For this review, take the finished solid that the model builds, in its own axes (mm). A direction names the side the tool comes from. Coordinates: 2 decimals unless noted, no trailing zeros. Loops run counter-clockwise (first coordinate to the right, second up) from the corner with the lowest first, then second, coordinate; pieces in that order, holes last. Notation, with made-up numbers: (37.25, -29.5) - (44.25, -29.5) arc R18 cw to (44.25, -3.5) - close; hole circle Ø7 at (47.5, 46). An arc over 180 degrees is marked (long way). Answer as a JSON object with one key per item and string values. Group by question number.
Item 1: To check wall thickness, follow line 1 (Y direction, x = 2, z = 1.5); line 2 (X direction, y = 2, z = -0.75); line 3 (Z direction, x = 0, y = 2). State the ranges of each line that lie inside material, in increasing order.
Item 2: We need section C-C (x = -5). Give the boundary of the cut face in (y, z), then the cut area to 3 significant figures.
Item 3: Clearance check with flat-ended pins moving along their axes: pin 1 (0.5 mm diameter, centred on x = 6, y = -3, fed in from +Z); pin 2 (1.8 mm diameter, centred on y = -1.5, z = 5.5, fed in from -X); pin 3 (2 mm diameter, centred on y = -2, z = -6.5, fed in from +X). State where each tip first meets the part, or that it passes through.
Item 4: We need section A-A (y = 2). Give the boundary of the cut face in (x, z), then the cut area to 3 significant figures.
Item 5: We need section D-D (y = -2.5). Give the boundary of the cut face in (x, z).
Item 6: We need section B-B (z = 0). Give the boundary of the cut face in (x, y), then the cut area to 3 significant figures.
Item 7: Mouldability with a two-part tool opening along X and no side actions: class faces 1 (the flat face through (-1.1, 0, -2.1)), 2 (the flat face through (4.6, -2, -1)), 3 (the flat face through (4.123, -2, -4)) as released by +X, released by -X, zero draft, split by the parting line, or undercut.
Item 8: Tool access review of faces 4 (the flat face through (7, -2, 1.002)), 5 (the flat face through (2, 3, 2)), 6 (the flat face through (-1, -3.5, 0)), 7 (the cylindrical face through (2.15, 1.48, 0.07)): name each direction out of +Z, -Z, +X, -X, +Y, -Y from which nothing blocks a thin tool from reaching the whole face with its end or side.
from build123d import *

# Parameters (mm, degrees)
SKETCH1_R           = 9
SKETCH1_R_2         = 2.6
BOSS_EXTRUDE1_DEPTH = 3
BOSS_EXTRUDE2_DEPTH = 3.5
SKETCH4_R           = 2.6
BOSS_EXTRUDE3_DEPTH = 3
CUT_EXTRUDE1_DEPTH  = 10


with BuildPart() as part:
    # Sketch1 → Boss-Extrude1 (new body)
    with BuildSketch(Plane(origin=(0, 0, 0), x_dir=(1, 0, 0), z_dir=(0, 1, 0))):
        Circle(SKETCH1_R)
        with Locations((-5, 0)):
            Circle(SKETCH1_R_2, mode=Mode.SUBTRACT)
        with BuildLine():
            Line((-1.54029218, 1.5), (-1.54029218, -1.5))
            ThreePointArc((-1.54029218, -1.5), (2.15, 0), (-1.54029218, 1.5))
        make_face(mode=Mode.SUBTRACT)
    extrude(amount=BOSS_EXTRUDE1_DEPTH)

    # Sketch2 → Boss-Extrude2 (add)
    with BuildSketch(Plane.XZ):
        with BuildLine():
            Line((4.123105626, 8), (4.123105626, -8))
            ThreePointArc((4.123105626, -8), (9, 0), (4.123105626, 8))
        make_face()
    extrude(amount=BOSS_EXTRUDE2_DEPTH)

    # Sketch4 → Boss-Extrude3 (add)
    with BuildSketch(Plane.XZ.offset(3.5)):
        with BuildLine():
            ThreePointArc((4.123105626, 8), (-9, 0), (4.123105626, -8))
            ThreePointArc((4.123105626, -8), (9, 0), (4.123105626, 8))
        make_face()
        with Locations((-5, 0)):
            Circle(SKETCH4_R, mode=Mode.SUBTRACT)
    extrude(amount=BOSS_EXTRUDE3_DEPTH)

    # Sketch5 → Cut-Extrude1 (cut)
    with BuildSketch(Plane(origin=(0, 3, 0), x_dir=(1, 0, 0), z_dir=(0, 1, 0))):
        Polygon((3.25, 0.798435283), (3.25, -1.001564717), (4.6, -1.001564717), (4.6, -2.351564717), (6.4, -2.351564717), (6.4, -1.001564717), (7.75, -1.001564717), (7.75, 0.798435283), (6.4, 0.798435283), (6.4, 2.148435283), (4.6, 2.148435283), (4.6, 0.798435283), align=None)
    extrude(amount=-CUT_EXTRUDE1_DEPTH, mode=Mode.SUBTRACT)


solid = part.part
Check sheet entries:
{
 "1": {"line 1": "y = -6.5 to -3.5, 0 to 3", "line 2": "x = -8.97 to -7.49, -2.51 to -1.54, 2.01 to 3.25, 7.75 to 8.97", "line 3": "z = -9 to -2.15, 2.15 to 9"},
 "2": {"outline": "(-6.5, -7.48) - (-3.5, -7.48) - (-3.5, -2.6) - (-6.5, -2.6) - close; (-6.5, 2.6) - (-3.5, 2.6) - (-3.5, 7.48) - (-6.5, 7.48) - close; (0, -7.48) - (3, -7.48) - (3, -2.6) - (0, -2.6) - close; (0, 2.6) - (3, 2.6) - (3, 7.48) - (0, 7.48) - close", "area": "58.6 mm2"},
 "3": {"pin 1": "stops at z = 6.92", "pin 2": "stops at x = 4.12", "pin 3": "stops at x = 7.12"},
 "4": {"outline": "circle Ø18 at (0, 0); hole circle Ø5.2 at (-5, 0); hole (-1.54, -1.5) arc R2.15 ccw (long way) to (-1.54, 1.5) - close; hole (3.25, -0.8) - (4.6, -0.8) - (4.6, -2.15) - (6.4, -2.15) - (6.4, -0.8) - (7.75, -0.8) - (7.75, 1) - (6.4, 1) - (6.4, 2.35) - (4.6, 2.35) - (4.6, 1) - (3.25, 1) - close", "area": "207 mm2"},
 "5": {"outline": "(4.12, -8) arc R9 ccw to (4.12, 8) - (4.12, 1) - (4.6, 1) - (4.6, 2.35) - (6.4, 2.35) - (6.4, 1) - (7.75, 1) - (7.75, -0.8) - (6.4, -0.8) - (6.4, -2.15) - (4.6, -2.15) - (4.6, -0.8) - (4.12, -0.8) - close"},
 "6": {"outline": "(-9, -6.5) - (-7.6, -6.5) - (-7.6, -3.5) - (-9, -3.5) - close; (-9, 0) - (-7.6, 0) - (-7.6, 3) - (-9, 3) - close; (-2.4, -6.5) - (3.25, -6.5) - (3.25, -3.5) - (-2.4, -3.5) - close; (-2.4, 0) - (-1.54, 0) - (-1.54, 3) - (-2.4, 3) - close; (2.15, 0) - (3.25, 0) - (3.25, 3) - (2.15, 3) - close; (7.75, -6.5) - (9, -6.5) - (9, 3) - (7.75, 3) - close", "area": "43.1 mm2"},
 "7": {"face 1": "zero draft", "face 2": "undercut", "face 3": "released by -X"},
 "8": {"face 4": "+Y, -Y", "face 5": "+Z, -Z, +X, -X, +Y", "face 6": "+Z, -Z, -X", "face 7": "+Y"}
}
